from build123d import *

# Parameters (mm, degrees)
F8_DEPTH  = 5
F9_DEPTH  = 5
F10_R     = 7.6519091013
F11_DEPTH = 99
F12_DEPTH = 15


with BuildPart() as f6:
    # F5 (on offset) → F6 (revolve)
    with BuildSketch(Plane(origin=(17.6776695297, 17.6776695297, 0), x_dir=(-0.7071067812, 0.7071067812, 0), z_dir=(0.7071067812, 0.7071067812, 0))):
        with BuildLine():
            Line((-82.2007035037, 49.919500947), (-75.3873662255, 49.919500947))
            Line((-75.3873662255, 49.919500947), (-11.9189445844, 49.919500947))
            Line((-11.9189445844, 49.919500947), (-11.9189445844, 55.2996545256))
            Line((-11.9189445844, 55.2996545256), (-25.3694628348, 58.2600160659))
            Line((-25.3694628348, 58.2600160659), (-29.349628467, 60.3313259006))
            Line((-29.349628467, 60.3313259006), (-41.0251509784, 60.3313259006))
            ThreePointArc((-41.0251509784, 60.3313259006), (-53.2737810815, 62.9286025134), (-65.5224111845, 60.3313259006))
            Line((-65.5224111845, 60.3313259006), (-73.8964080811, 62.7087488713))
            Line((-73.8964080811, 62.7087488713), (-73.8964080811, 68.3596432209))
            ThreePointArc((-73.8964080811, 68.3596432209), (-80.0288579522, 60.031377251), (-82.2007035037, 49.919500947))
        make_face()
    revolve(axis=Axis((48.5451117367, -13.1897726774, 49.919500947), (-0.7071067812, 0.7071067812, 0)))

    # F7 (on offset) → F8 (join)
    with BuildSketch(Plane(origin=(17.6776695297, 17.6776695297, 0), x_dir=(-0.7071067812, 0.7071067812, 0), z_dir=(0.7071067812, 0.7071067812, 0))):
        Polygon((2.3306398652, 52.3042623256), (-12.1975196525, 57.7270142357), (-12.1975196525, 41.5063718017), (2.3306398652, 45.2429535571), align=None)
    extrude(amount=F8_DEPTH)

    # F7 (on offset) → F9 (join)
    with BuildSketch(Plane(origin=(17.6776695297, 17.6776695297, 0), x_dir=(-0.7071067812, 0.7071067812, 0), z_dir=(0.7071067812, 0.7071067812, 0))):
        Polygon((2.3306398652, 52.3042623256), (-12.1975196525, 57.7270142357), (-12.1975196525, 41.5063718017), (2.3306398652, 45.2429535571), align=None)
    extrude(amount=-F9_DEPTH)

    # F10 (on offset) → F11 (join)
    with BuildSketch(Plane.XY.offset(-36)):
        with Locations((55.5105434031, -20.1552043437)):
            Circle(F10_R)
    extrude(amount=F11_DEPTH)

    # F10 (on offset) → F12 (join)
    with BuildSketch(Plane.XY.offset(-36)):
        with Locations((55.5105434031, -20.1552043437)):
            Circle(F10_R)
    extrude(amount=-F12_DEPTH)


solid = f6.part
Source: CAD feature listing. Evaluate the final solid. Frame: model axes, mm. A direction names the side the tool comes from. Give positions to 0.01 mm unless a question says otherwise; leave off trailing zeros. Write each loop counter-clockwise with the first axis right and the second up, starting at its lowest first coordinate (ties: lowest second). Pieces come first, ordered by that corner, then holes. Notation, with made-up numbers: (29.5, 17.5) -> (88.5, 17.5) arc R12 ccw to (88.5, 24.5) -> close; hole circle Ø10 at (-19.75, -33). An arc over 180 degrees is marked (long way). Return JSON: item names as keys, results as strings. Group by question number.
1. Section B-B, the plane z = 0.5. Output: boundary loops of the cut face in (x, y).
2. Access query for faces 4 (the face through (39.84, 3.611, 43.677)), 5 (the face through (62.579, -23.086, 61.986)), 6 (the face through (26.35, 9.1, 43.29)). Directions: +Z, -Z, +X, -X, +Y, -Y. A direction counts if a zero-diameter tool reaches every point of the face in a straight line with its end or side. Return the directions, or none.
3. Pin query (flat end, axial travel): pin 1 Ø4.5 at (x, y) = (52.5, -22.5) entering from +Z; pin 2 Ø8 at (y, z) = (-19.5, -5.5) entering from +X; pin 3 Ø10 at (y, z) = (-5, -3) entering from +X; pin 4 Ø8 at (y, z) = (-13.5, 4) entering from +X. Return the tip coordinate at first contact, or that it passes through.
4. Mould query, pull axis X, two halves, no side actions, for faces 1 (the face through (55, -20, -51)), 2 (the face through (21.144, 14.311, 54.978)), 3 (the face through (67.215, -37.29, 62.471)). Classes: +X half, -X half, draft (parallel to the pull), parting line (faces both ways), or undercut.
5. Material intervals for line 1 (Y direction, x = 55, z = 1.5); line 2 (Y direction, x = 60, z = 49); line 3 (X direction, y = -17, z = 33), sorted ascending. Write a range as from..to.
6. Section A-A, the plane x = 17.5. Output: boundary loops of the cut face in (y, z), then the cut area to 3 significant figures.
Determined:
{
 "1": {"outline": "circle Ø15.3 at (55.51, -20.16)"},
 "2": {"face 4": "none", "face 5": "+Z", "face 6": "-Z"},
 "3": {"pin 1": "stops at z = 63", "pin 2": "stops at x = 63.16", "pin 3": "passes through", "pin 4": "stops at x = 62.69"},
 "4": {"face 1": "draft", "face 2": "-X half", "face 3": "undercut"},
 "5": {"line 1": "y = -27.79..-12.52", "line 2": "y = -47.59..-44.51, -41.96..-7.1", "line 3": "x = 48.54..62.48"},
 "6": {"outline": "(10.78, 43.42) -> (20.8, 45.24) -> (20.8, 52.3) -> (10.78, 54.95) -> close", "area": "93.0 mm2"}
}
